```python
from build123d import *

# Parameters (mm, degrees)
SKETCH1_R            = 4.14655
BOSS_EXTRUDE1_DEPTH  = 3.048
FILLET1_R            = 12.7
CUT_EXTRUDE1_DEPTH   = 98.209690942
FILLET2_R            = 5.08
FILLET2_OF_MIRROR1_R = 5.08
BOSS_EXTRUDE2_DEPTH  = 3.048
FILLET3_R            = 7.62


with BuildPart() as part:
    # Sketch1 → Boss-Extrude1 (new body)
    with BuildSketch(Plane.XY):
        with BuildLine():
            Line((51.054, 0), (-51.054, 0))
            Line((-51.054, 0), (-51.054, -3.048))
            Line((-51.054, -3.048), (-63.754, -3.048))
            Line((-63.754, -3.048), (-63.754, 0))
            Line((-63.754, 0), (-76.901088515, 0))
            ThreePointArc((-76.901088515, 0), (-78.697139739, 0.743948776), (-79.441088515, 2.54))
            Line((-79.441088515, 2.54), (-79.441088515, 6.096))
            Line((-79.441088515, 6.096), (-82.489088515, 6.096))
            Line((-82.489088515, 6.096), (-82.489088515, 18.796))
            Line((-82.489088515, 18.796), (-79.441088515, 18.796))
            Line((-79.441088515, 18.796), (-50.69543442, 47.292942568))
            ThreePointArc((-50.69543442, 47.292942568), (-41.155344062, 51.338715816), (-31.452840209, 47.699619198))
            Line((-31.452840209, 47.699619198), (0, 19.05))
            Line((0, 19.05), (31.452840209, 47.699619198))
            ThreePointArc((31.452840209, 47.699619198), (41.155344062, 51.338715816), (50.69543442, 47.292942568))
            Line((50.69543442, 47.292942568), (79.441088515, 18.796))
            Line((79.441088515, 18.796), (82.489088515, 18.796))
            Line((82.489088515, 18.796), (82.489088515, 6.096))
            Line((82.489088515, 6.096), (79.441088515, 6.096))
            Line((79.441088515, 6.096), (79.441088515, 2.54))
            ThreePointArc((79.441088515, 2.54), (78.697139739, 0.743948776), (76.901088515, 0))
            Line((76.901088515, 0), (63.754, 0))
            Line((63.754, 0), (63.754, -3.048))
            Line((63.754, -3.048), (51.054, -3.048))
            Line((51.054, -3.048), (51.054, 0))
        make_face()
        with Locations((40.860165351, 37.371834649)):
            Circle(SKETCH1_R, mode=Mode.SUBTRACT)
        with Locations((-40.860165351, 37.371834649)):
            Circle(SKETCH1_R, mode=Mode.SUBTRACT)
    extrude(amount=-BOSS_EXTRUDE1_DEPTH)

    # Fillet1
    fillet1_edges = [part.edges().sort_by_distance(p)[0] for p in [
        (0, 19.05, -1.524),
    ]]
    fillet(fillet1_edges, radius=FILLET1_R)

    # Sketch3 → Cut-Extrude1 (cut, symmetric)
    with BuildSketch(Plane.XY):
        with BuildLine():
            Line((-49.43113261, 24.225449161), (-66.181508428, 7.62))
            Line((-66.181508428, 7.62), (-21.667355118, 7.62))
            Line((-21.667355118, 7.62), (-21.667355118, 15.24))
            Line((-21.667355118, 15.24), (-31.937865146, 24.595155188))
            ThreePointArc((-31.937865146, 24.595155188), (-40.758323194, 27.903424841), (-49.43113261, 24.225449161))
        make_face()
    cut_extrude1 = extrude(amount=CUT_EXTRUDE1_DEPTH, both=True, mode=Mode.SUBTRACT)

    # Fillet2
    fillet2_edges = [part.edges().sort_by_distance(p)[0] for p in [
        (-21.667355118, 7.62, -1.524),
        (-66.181508428, 7.62, -1.524),
        (-21.667355118, 15.24, -1.524),
    ]]
    fillet(fillet2_edges, radius=FILLET2_R)

    # Mirror1: Cut-Extrude1 across plane
    add(cut_extrude1.mirror(Plane(origin=(0, 0, 0), x_dir=(0, 0, 1), z_dir=(1, 0, 0))), mode=Mode.SUBTRACT)

    # Fillet2 of Mirror1
    fillet2_of_mirror1_edges = [part.edges().sort_by_distance(p)[0] for p in [
        (21.667355118, 7.62, -1.524),
        (66.181508428, 7.62, -1.524),
        (21.667355118, 15.24, -1.524),
    ]]
    fillet(fillet2_of_mirror1_edges, radius=FILLET2_OF_MIRROR1_R)

    # Sketch4 → Boss-Extrude2 (add)
    with BuildSketch(Plane(origin=(0, 0, -3.048), x_dir=(-1, 0, 0), z_dir=(0, 0, -1))):
        Polygon((-82.489088515, 70.358), (-79.441088515, 70.358), (-53.661061877, 44.352974145), (-60.010822133, 38.058152927), (-79.441088515, 57.658), (-82.489088515, 57.658), align=None)
    boss_extrude2 = extrude(amount=-BOSS_EXTRUDE2_DEPTH)

    # Mirror3: Boss-Extrude2 across plane
    add(boss_extrude2.mirror(Plane(origin=(0, 0, 0), x_dir=(0, 0, 1), z_dir=(1, 0, 0))))

    # Fillet3
    fillet3_edges = [part.edges().sort_by_distance(p)[0] for p in [
        (60.010822133, 38.058152927, -1.524),
        (53.661061877, 44.352974145, -1.524),
        (-60.010822133, 38.058152927, -1.524),
        (-53.661061877, 44.352974145, -1.524),
    ]]
    fillet(fillet3_edges, radius=FILLET3_R)


solid = part.part
```
Could you check a few things on this model? Use its own coordinates, in mm. A direction names the side the tool comes from. Give positions to 0.01 mm unless a question says otherwise; leave off trailing zeros. Write each loop counter-clockwise with the first axis right and the second up, starting at its lowest first coordinate (ties: lowest second). Pieces come first, ordered by that corner, then holes. Notation, with made-up numbers: (59, 79) - (116, 79) arc R22 ccw to (116, 104) - close; hole circle Ø6 at (55, -17). An arc over 180 degrees is marked (long way). One line per item, written item: value. Start each with the question number.
Item 1: Imagine slicing it at A-A, the plane x = 40. List the corners of the cut face in (y, z) for me, and give its area (3 significant figures).
Item 2: Imagine slicing it at D-D, the plane x = -61.5. List the corners of the cut face in (y, z) for me.
Item 3: Imagine slicing it at C-C, the plane x = 11.5. List the corners of the cut face in (y, z) for me.
Item 4: Please list where these lines run through material, in increasing order: line 1 (Y direction, x = -39, z = -2.3); line 2 (X direction, y = 11, z = -1.65); line 3 (X direction, y = 36, z = -2.7). Write a range as from..to.
Item 5: I'm going to push flat-ended pins straight in: pin 1 (1.5 mm diameter, centred on y = -2, z = -1, fed in from -X); pin 2 (1.5 mm diameter, centred on x = -81, z = -2, fed in from -Y); pin 3 (1.5 mm diameter, centred on x = -61, z = -0.5, fed in from +Y). Where does each tip first touch, or does it pass through?
Item 6: If we mould it in two halves opening along X, with no side actions, what happens to faces 1 (the face through (58.506, 10.689, -1.503)), 2 (the face through (81, 6.096, -2)), 3 (the face through (72.334, 25.842, -1.503))? For each: +X half, -X half, draft (parallel to the pull), parting line (faces both ways), or undercut.
Item 7: Which directions (+Z, -Z, +X, -X, +Y, -Y) give clear straight access to the entire face, cutting with the end or side of a thin tool? Please do faces 4 (the face through (-69.28, 60.11, -1.55)), 5 (the face through (-81, 57.658, -2)), 6 (the face through (40.623, 27.906, -1.503)).
Item 8: Imagine slicing it at B-B, the plane z = -1.3. Give the number of separate pieces and of enclosed holes in the cut face, and give its area (3 significant figures).
Geometry says:
1. outline: (0, -3.05) - (7.62, -3.05) - (7.62, 0) - (0, 0) - close; (27.9, -3.05) - (33.32, -3.05) - (33.32, 0) - (27.9, 0) - close; (41.43, -3.05) - (51.32, -3.05) - (51.32, 0) - (41.43, 0) - close
1. area: 69.9 mm^2
2. outline: (-3.05, -3.05) - (52.26, -3.05) - (52.26, 0) - (-3.05, 0) - close
3. outline: (0, -3.05) - (29.53, -3.05) - (29.53, 0) - (0, 0) - close
4. line 1: 0..7.62, 27.82..33.67, 41.08..51.22
4. line 2: -82.49..-58.63, -21.96..21.96, 58.63..82.49
4. line 3: -63.46..-44.77, -36.95..-18.61, 18.61..36.95, 44.77..63.46
5. pin 1: x = -63.75
5. pin 2: y = 6.1
5. pin 3: y = 52.51
6. face 1: undercut
6. face 2: draft
6. face 3: +X half
7. face 4: +Z, -Z, +Y
7. face 5: +Z, -Z, -X
7. face 6: +Z, -Z
8. separate pieces: 1
8. enclosed holes: 4
8. area: 5,570 mm^2
